Build history of the part. All positions in model axes, mm. A direction names the side the tool comes from. Round coordinates to 2 decimals unless told otherwise and drop trailing zeros. Write each loop counter-clockwise with the first axis right and the second up, starting at its lowest first coordinate (ties: lowest second). Pieces come first, ordered by that corner, then holes.
1) Saw through at B-B (y = 49.5). Write the cut outline in (x, z).
2) Flat gauge pins, fed straight in: pin 1 (1.1 mm diameter, centred on y = 20, z = -5, fed in from +X); pin 2 (20 mm diameter, centred on x = 0.5, y = 13.5, fed in from +Z); pin 3 (3 mm diameter, centred on x = -24, z = -0.5, fed in from -Y). Where does each tip first touch, or does it go through?
3) Wall check: probe 1 along Z at (x, y) = (-66.5, -44); probe 2 along Y at (x, z) = (-63, -9.5); probe 3 along Y at (x, z) = (0, 0.35) (3 decimals). Give the ranges that are in metal, low to high.
4) Pull direction Z, two halves, no side cores. Call faces 1 (the cylindrical face through (-27.105, -26.74, -9.493)), 2 (the flat face through (26, -26, 0)), 3 (the flat face through (0, 7, -5.5)): +Z half, -Z half, draft (parallel to the pull), parting line (faces both ways), or undercut.
5) Saw through at C-C (z = -7.25). Write the cut outline in (x, y) (3 decimals).
6) Saw through at A-A (x = 0). Write the cut outline in (y, z) (3 decimals).
7) Which spindle directions (+Z, -Z, +X, -X, +Y, -Y) get a long thin tool onto all of the face, cutting with end or side? Do faces 4 (the cylindrical face through (55.263, -56.313, 0.493)), 5 (the flat face through (33, -6, -10)). Say none if no direction does.
8) Saw through at D-D (x = -22). State how many separate pieces and enclosed holes the cut face has, plus the area to 3 significant figures.
from build123d import *

# Parameters (mm, degrees)
SKETCH1_R           = 88.9
SKETCH1_R_2         = 33.075
BOSS_EXTRUDE1_DEPTH = 1
SKETCH2_R           = 36.075
SKETCH2_R_2         = 33.075
BOSS_EXTRUDE2_DEPTH = 3.5
SKETCH3_R           = 36.075
SKETCH3_R_2         = 33.075
SKETCH3_R_3         = 5
BOSS_EXTRUDE3_DEPTH = 1


with BuildPart() as part:
    # Sketch1 → Boss-Extrude1 (new body)
    with BuildSketch(Plane.XY):
        Circle(SKETCH1_R)
        Circle(SKETCH1_R_2, mode=Mode.SUBTRACT)
        with BuildLine():
            Line((-6.699774442, 76.240588003), (-9.885609858, 38.107539665))
            ThreePointArc((-9.885609858, 38.107539665), (-10.319263885, 37.02174666), (-11.285844597, 36.363929061))
            ThreePointArc((-11.285844597, 36.363929061), (-26.923090694, 26.923090694), (-36.363929061, 11.285844597))
            ThreePointArc((-36.363929061, 11.285844597), (-37.02174666, 10.319263885), (-38.107539665, 9.885609858))
            Line((-38.107539665, 9.885609858), (-76.240588003, 6.699774442))
            ThreePointArc((-76.240588003, 6.699774442), (-77.842317358, 7.299939499), (-78.39427914, 8.918912388))
            ThreePointArc((-78.39427914, 8.918912388), (-55.790725036, 55.790725036), (-8.918912388, 78.39427914))
            ThreePointArc((-8.918912388, 78.39427914), (-7.299939499, 77.842317358), (-6.699774442, 76.240588003))
        make_face(mode=Mode.SUBTRACT)
        with BuildLine():
            Line((6.699774442, 76.240588003), (9.885609858, 38.107539665))
            ThreePointArc((9.885609858, 38.107539665), (10.319263885, 37.02174666), (11.285844597, 36.363929061))
            ThreePointArc((11.285844597, 36.363929061), (26.923090694, 26.923090694), (36.363929061, 11.285844597))
            ThreePointArc((36.363929061, 11.285844597), (37.02174666, 10.319263885), (38.107539665, 9.885609858))
            Line((38.107539665, 9.885609858), (76.240588003, 6.699774442))
            ThreePointArc((76.240588003, 6.699774442), (77.842317358, 7.299939499), (78.39427914, 8.918912388))
            ThreePointArc((78.39427914, 8.918912388), (55.790725036, 55.790725036), (8.918912388, 78.39427914))
            ThreePointArc((8.918912388, 78.39427914), (7.299939499, 77.842317358), (6.699774442, 76.240588003))
        make_face(mode=Mode.SUBTRACT)
        with BuildLine():
            Line((76.240588003, -6.699774442), (38.107539665, -9.885609858))
            ThreePointArc((38.107539665, -9.885609858), (37.02174666, -10.319263885), (36.363929061, -11.285844597))
            ThreePointArc((36.363929061, -11.285844597), (26.923090694, -26.923090694), (11.285844597, -36.363929061))
            ThreePointArc((11.285844597, -36.363929061), (10.319263885, -37.02174666), (9.885609858, -38.107539665))
            Line((9.885609858, -38.107539665), (6.699774442, -76.240588003))
            ThreePointArc((6.699774442, -76.240588003), (7.299939499, -77.842317358), (8.918912388, -78.39427914))
            ThreePointArc((8.918912388, -78.39427914), (55.790725036, -55.790725036), (78.39427914, -8.918912388))
            ThreePointArc((78.39427914, -8.918912388), (77.842317358, -7.299939499), (76.240588003, -6.699774442))
        make_face(mode=Mode.SUBTRACT)
        with BuildLine():
            Line((-9.885609858, -38.107539665), (-6.699774442, -76.240588003))
            ThreePointArc((-6.699774442, -76.240588003), (-7.299939499, -77.842317358), (-8.918912388, -78.39427914))
            ThreePointArc((-8.918912388, -78.39427914), (-55.790725036, -55.790725036), (-78.39427914, -8.918912388))
            ThreePointArc((-78.39427914, -8.918912388), (-77.842317358, -7.299939499), (-76.240588003, -6.699774442))
            Line((-76.240588003, -6.699774442), (-38.107539665, -9.885609858))
            ThreePointArc((-38.107539665, -9.885609858), (-37.02174666, -10.319263885), (-36.363929061, -11.285844597))
            ThreePointArc((-36.363929061, -11.285844597), (-26.923090694, -26.923090694), (-11.285844597, -36.363929061))
            ThreePointArc((-11.285844597, -36.363929061), (-10.319263885, -37.02174666), (-9.885609858, -38.107539665))
        make_face(mode=Mode.SUBTRACT)
    extrude(amount=BOSS_EXTRUDE1_DEPTH)

    # Sketch2 → Boss-Extrude2 (add)
    with BuildSketch(Plane(origin=(0, 0, 0), x_dir=(-1, 0, 0), z_dir=(0, 0, -1))):
        with Locations(Location((0, 0, 0), (0, 0, 180))):
            Circle(SKETCH2_R)
        Circle(SKETCH2_R_2, mode=Mode.SUBTRACT)
    extrude(amount=BOSS_EXTRUDE2_DEPTH)

    # Sketch3 → Boss-Extrude3 (add)
    with BuildSketch(Plane(origin=(0, 0, -3.5), x_dir=(-1, 0, 0), z_dir=(0, 0, -1))):
        with Locations(Location((0, 0, 0), (0, 0, 180))):
            Circle(SKETCH3_R)
        with Locations(Location((0, 0, 0), (0, 0, 4.334881134))):
            Circle(SKETCH3_R_2, mode=Mode.SUBTRACT)
        with BuildLine():
            Line((-2.5, 11.736694594), (-2.5, 32.980382427))
            ThreePointArc((-2.5, 32.980382427), (-23.387556788, 23.387556788), (-32.980382427, 2.5))
            Line((-32.980382427, 2.5), (-11.736694594, 2.5))
            ThreePointArc((-11.736694594, 2.5), (-12, 0), (-11.736694594, -2.5))
            Line((-11.736694594, -2.5), (-32.980382427, -2.5))
            ThreePointArc((-32.980382427, -2.5), (-23.387556788, -23.387556788), (-2.5, -32.980382427))
            Line((-2.5, -32.980382427), (-2.5, -11.736694594))
            ThreePointArc((-2.5, -11.736694594), (0, -12), (2.5, -11.736694594))
            Line((2.5, -11.736694594), (2.5, -32.980382427))
            ThreePointArc((2.5, -32.980382427), (23.387556788, -23.387556788), (32.980382427, -2.5))
            Line((32.980382427, -2.5), (11.736694594, -2.5))
            ThreePointArc((11.736694594, -2.5), (12, 0), (11.736694594, 2.5))
            Line((11.736694594, 2.5), (32.980382427, 2.5))
            ThreePointArc((32.980382427, 2.5), (23.387556788, 23.387556788), (2.5, 32.980382427))
            Line((2.5, 32.980382427), (2.5, 11.736694594))
            ThreePointArc((2.5, 11.736694594), (0, 12), (-2.5, 11.736694594))
        make_face()
        with Locations((-15.496643432, 15.496643432)):
            Circle(SKETCH3_R_3, mode=Mode.SUBTRACT)
        with BuildLine():
            ThreePointArc((-5.837165408, -2.5), (-6.35, 0), (-5.837165408, 2.5))
            ThreePointArc((-5.837165408, 2.5), (-4.490128061, 4.490128061), (-2.5, 5.837165408))
            ThreePointArc((-2.5, 5.837165408), (0, 6.35), (2.5, 5.837165408))
            ThreePointArc((2.5, 5.837165408), (4.490128061, 4.490128061), (5.837165408, 2.5))
            ThreePointArc((5.837165408, 2.5), (6.220470253, 1.27602893), (6.35, 0))
            ThreePointArc((6.35, 0), (6.220470253, -1.27602893), (5.837165408, -2.5))
            ThreePointArc((5.837165408, -2.5), (4.490128061, -4.490128061), (2.5, -5.837165408))
            ThreePointArc((2.5, -5.837165408), (0, -6.35), (-2.5, -5.837165408))
            ThreePointArc((-2.5, -5.837165408), (-4.490128061, -4.490128061), (-5.837165408, -2.5))
        make_face(mode=Mode.SUBTRACT)
    extrude(amount=BOSS_EXTRUDE3_DEPTH)

    # Mirror4: part across plane


with BuildPart() as part_1:
    add(part.part)
    add(part.part.mirror(Plane(origin=(-79.506421356, 0, -4.5), x_dir=(1, 0, 0), z_dir=(0, 0, -1))))


solid = part_1.part
Evaluation:
1. outline: (-73.84, -10) - (-61.44, -10) - (-61.44, -9) - (-73.84, -9) - close; (-73.84, 0) - (-61.44, 0) - (-61.44, 1) - (-73.84, 1) - close; (-8.93, -10) - (8.93, -10) - (8.93, -9) - (-8.93, -9) - close; (-8.93, 0) - (8.93, 0) - (8.93, 1) - (-8.93, 1) - close; (61.44, -10) - (73.84, -10) - (73.84, -9) - (61.44, -9) - close; (61.44, 0) - (73.84, 0) - (73.84, 1) - (61.44, 1) - close
2. pin 1: stops at x = 30.38
2. pin 2: stops at z = -3.5
2. pin 3: stops at y = -85.98
3. probe 1: z = -10 to -9, 0 to 1
3. probe 2: y = -62.72 to -47.5, -7.81 to 7.81, 47.5 to 62.72
3. probe 3: y = -88.9 to -33.075, 33.075 to 88.9
4. face 1: draft
4. face 2: undercut
4. face 3: -Z half
5. outline: circle Ø72.15 at (0, 0); hole circle Ø66.15 at (0, 0)
6. outline: (-88.9, -10) - (-33.075, -10) - (-33.075, 1) - (-88.9, 1) - (-88.9, 0) - (-36.075, 0) - (-36.075, -9) - (-88.9, -9) - close; (-12, -5.5) - (-6.35, -5.5) - (-6.35, -3.5) - (-12, -3.5) - close; (6.35, -5.5) - (12, -5.5) - (12, -3.5) - (6.35, -3.5) - close; (33.075, -10) - (88.9, -10) - (88.9, -9) - (36.075, -9) - (36.075, 0) - (88.9, 0) - (88.9, 1) - (33.075, 1) - close
7. face 4: +Z, -Z
7. face 5: -Z, +X, -X, +Y, -Y
8. separate pieces: 6
8. enclosed holes: 0
8. area: 226 mm2
